Verification items for the finished model (mm, model axes). Round coordinates to 2 decimals unless told otherwise and drop trailing zeros. Order: outer loops, then holes, each group sorted by start corner. A loop starts at its lowest first (then second) coordinate and runs counter-clockwise, first axis right, second up. Notation, with made-up numbers: (49, 61) -> (105, 61) arc R33 cw to (105, 100) -> close; hole circle Ø7 at (53, 12). An arc over 180 degrees is marked (long way). Write item = value, one per line. Start each with the question number.
from build123d import *

# Parameters (mm, degrees)
F0_R      = 14.2748
F0_R_2    = 12.827
F1_DEPTH  = 266.7
F3_DEPTH  = 12.7
F4_R      = 14.2748
F4_R_2    = 12.827
F5_DEPTH  = 76.2
F7_R      = 1.524
F8_DEPTH  = 5.08
F10_R     = 1.5875
F11_DEPTH = 5.08
F12_R     = 14.2875
F13_DEPTH = 256.54
F14_R     = 14.2748
F14_R_2   = 12.827
F15_DEPTH = 3.81
F16_R     = 14.2748
F16_R_2   = 10.795
F17_DEPTH = 102.87
F18_DEPTH = 74.93


with BuildPart() as f1:
    # F0 (on Top) → F1 (new body)
    with BuildSketch(Plane.XY):
        Circle(F0_R)
        Circle(F0_R_2, mode=Mode.SUBTRACT)
    extrude(amount=F1_DEPTH)

    # F2 (on face) → F3 (join)
    with BuildSketch(Plane.XY.offset(266.7)):
        with BuildLine():
            Line((-3.175, 12.4278438999), (-3.175, 13.9172299701))
            ThreePointArc((-3.175, 13.9172299701), (0, -14.2748), (3.175, 13.9172299701))
            Line((3.175, 13.9172299701), (3.175, 12.4278438999))
            ThreePointArc((3.175, 12.4278438999), (0, -12.827), (-3.175, 12.4278438999))
        make_face()
    extrude(amount=F3_DEPTH)

    # F4 (on face) → F5 (join)
    with BuildSketch(Plane.XY.offset(279.4)):
        Circle(F4_R)
        Circle(F4_R_2, mode=Mode.SUBTRACT)
    extrude(amount=F5_DEPTH)

    # F7 (on offset) → F8 (join)
    with BuildSketch(Plane.YZ.offset(12.827)):
        with Locations((0, 12.7)):
            Circle(F7_R)
    extrude(amount=F8_DEPTH)

    # F10 (on offset) → F11 (join)
    with BuildSketch(Plane.YZ.offset(-12.827)):
        with Locations((0, 12.7)):
            Circle(F10_R)
    extrude(amount=-F11_DEPTH)

    # F12 (on face) → F13 (cut)
    with BuildSketch(Plane.XY.offset(355.6)):
        Circle(F12_R)
    extrude(amount=-F13_DEPTH, mode=Mode.SUBTRACT)

    # F14 (on face) → F15 (join)
    with BuildSketch(Plane(origin=(0, 0, 0), x_dir=(1, 0, 0), z_dir=(0, 0, -1))):
        Circle(F14_R)
        Circle(F14_R_2, mode=Mode.SUBTRACT)
    extrude(amount=F15_DEPTH)

    # F16 (on face) → F17 (join)
    with BuildSketch(Plane.XY.offset(99.06)):
        Circle(F16_R)
        Circle(F16_R_2, mode=Mode.SUBTRACT)
    extrude(amount=-F17_DEPTH)

    # F16 (on face) → F18 (join)
    with BuildSketch(Plane.XY.offset(99.06)):
        Circle(F16_R)
        Circle(F16_R_2, mode=Mode.SUBTRACT)
    extrude(amount=F18_DEPTH)

    # F19: F1 across face


with BuildPart() as f1_1:
    add(f1.part)
    add(f1.part.mirror(Plane.XY.offset(173.99)))


solid = f1_1.part
(1) Depth check by flat-ended pin: pin 1 (8 mm diameter, centred on x = -9, z = 123.5, fed in from +Y); pin 2 (3 mm diameter, centred on x = 3, z = 256.5, fed in from -Y); pin 3 (4 mm diameter, centred on x = 9.5, y = -1, fed in from +Z); pin 4 (1 mm diameter, centred on y = 0.5, z = 121.5, fed in from -X). Enter the tip coordinate at first touch or a pass-through.
(2) Cross-section at C-C (z = 47). Enter the section's corners in (x, y) (3 decimals).
(3) Cross-section at B-B (y = -7.25). Enter the section's corners in (x, z).
(4) Cross-section at A-A (x = 0). Enter the section's corners in (y, z) (3 decimals).
(5) Scan lines: line 1 along Y through (x, z) = (0, 269) (3 decimals); line 2 along X through (y, z) = (-3.5, 185); line 3 along Y through (x, z) = (-6.5, 23). Record each from-to range of solid material in increasing order. Write a range as from..to.
Outcome:
q1.pin_1 = 13.37
q1.pin_2 = -14.2
q1.pin_3 = 351.79
q1.pin_4 = -14.27
q2.outline = circle Ø28.55 at (0, 0); hole circle Ø21.59 at (0, 0)
q3.outline = (-12.3, -3.81) -> (-8, -3.81) -> (-8, 351.79) -> (-12.3, 351.79) -> close; (8, -3.81) -> (12.3, -3.81) -> (12.3, 351.79) -> (8, 351.79) -> close
q4.outline = (-14.275, -3.81) -> (-10.795, -3.81) -> (-10.795, 351.79) -> (-14.275, 351.79) -> close; (10.795, -3.81) -> (14.275, -3.81) -> (14.275, 351.79) -> (10.795, 351.79) -> close
q5.line_1 = -14.275..-10.795, 10.795..14.275
q5.line_2 = -13.84..-10.21, 10.21..13.84
q5.line_3 = -12.71..-8.62, 8.62..12.71
